from build123d import *

# Parameters (mm, degrees)
SKETCH1_W                  = 3
SKETCH1_H                  = 65
CUT_EXTRUDE1_DEPTH         = 66.138314378
CUT_EXTRUDE1_DEPTH_BACK    = 66.138314378
SKETCH2_R                  = 1.55
M3X0_5_TAPPED_HOLE1_REACH  = 67.138
M3X0_5_TAPPED_HOLE1_BORE_R = 1.25
CHAMFER1_SIZE              = 1
CHAMFER1_SIZE2             = 0.363970234


with BuildPart() as part:
    # Sketch1 → Revolve1 (revolve)
    with BuildSketch(Plane.XY, mode=Mode.PRIVATE) as revolve1_sk:
        with Locations((1.5, 32.5)):
            Rectangle(SKETCH1_W, SKETCH1_H)
    revolve(revolve1_sk.sketch.rotate(Axis((0, -5.428885746, 0), (0, 1, 0)), 90), axis=Axis((0, -5.428885746, 0), (0, 1, 0)))

    # Sketch2 → Cut-Extrude1 (cut, two sides: drawn at the far end of the back side and taken through both)
    with BuildSketch(Plane(origin=(0, 0, 0), x_dir=(0, 0, -1), z_dir=(1, 0, 0)).offset(-CUT_EXTRUDE1_DEPTH_BACK)):
        with Locations((0, 59)):
            Circle(SKETCH2_R)
    extrude(amount=CUT_EXTRUDE1_DEPTH + CUT_EXTRUDE1_DEPTH_BACK, mode=Mode.SUBTRACT)

    # M3x0.5 Tapped Hole1 bore → M3x0.5 Tapped Hole1 (cut, up to next)
    with BuildSketch(Plane(origin=(0, 65, 0), x_dir=(-1, 0, 0), z_dir=(0, 1, 0)), mode=Mode.PRIVATE) as m3x0_5_tapped_hole1_sk1:
        Circle(M3X0_5_TAPPED_HOLE1_BORE_R)
    m3x0_5_tapped_hole1_tool1 = extrude(m3x0_5_tapped_hole1_sk1.sketch, amount=-M3X0_5_TAPPED_HOLE1_REACH, mode=Mode.PRIVATE) & part.part
    add(m3x0_5_tapped_hole1_tool1.solids().sort_by_distance((0, 65, 0))[0], mode=Mode.SUBTRACT)

    # Chamfer1
    chamfer1_edges = [part.edges().sort_by_distance(p)[0] for p in [
        (0, 0, 3),
    ]]
    chamfer1_side = [part.faces().sort_by_distance(p)[0] for p in [
        (0, 32.5, 3),
    ]]
    chamfer(chamfer1_edges, length=CHAMFER1_SIZE, length2=CHAMFER1_SIZE2, reference=chamfer1_side[0])


solid = part.part
CAD build for the part. Positions are in the model's coordinates, mm. A direction names the side the tool comes from. Give positions to 0.01 mm unless a question says otherwise; leave off trailing zeros. Write each loop counter-clockwise with the first axis right and the second up, starting at its lowest first coordinate (ties: lowest second). Pieces come first, ordered by that corner, then holes. Notation, with made-up numbers: M -3,-23 L 32,-23 A19 ccw 32,7 Z; hole C 10.5,-22 d3. An arc over 180 degrees is marked long. Put each result on its own line as item: value. Start each with the question number.
(1) Probe L1, parallel to X at y = 60.9, z = 0; L2, parallel to Z at x = -0.25, y = 59; L3, parallel to Z at x = 1.25, y = 59. List the from-to ranges inside material, lowest first.
(2) Band-saw the part on C-C, the plane y = 59. Write the cut outline in (x, z), and give its area (3 significant figures).
(3) Which spindle directions (+Z, -Z, +X, -X, +Y, -Y) get a long thin tool onto all of the face, cutting with end or side? Do faces 1 (the face through (0, 0, 0)), 2 (the face through (-1.19, 62.49, 0.38)). Say none if no direction does.
(4) Band-saw the part on D-D, the plane y = 22.5. Write the cut outline in (x, z), and give its area (3 significant figures).
(5) Mould opens along Z. For faces 3 (the face through (-0.042, 57.487, 0.336)), 4 (the face through (1, 65, 1)), 5 (the face through (-0.9, 33.45, -2.86)) say: +Z half, -Z half, draft (parallel to the pull), parting line (faces both ways), or undercut.
(6) Band-saw the part on A-A, the plane z = 0. Write the cut outline in (x, y), and give its area (3 significant figures).
(7) Flat gauge pins, fed straight in: pin 1 Ø1.5 at (y, z) = (28.5, 1) entering from +X; pin 2 Ø2 at (x, y) = (-1.5, 18) entering from +Z. Where does each tip first touch, or does it go through?
(8) Band-saw the part on B-B, the plane x = 0. Write the cut outline in (y, z).
Response values:
1. L1: x = -3 to -1.25, 1.25 to 3
1. L2: z = -2.99 to -1.55, 1.55 to 2.99
1. L3: z = -2.73 to -1.55, 1.55 to 2.73
2. outline: M -2.57,-1.55 A3 ccw 2.57,-1.55 Z; M -2.57,1.55 L 2.57,1.55 A3 ccw Z
2. area: 10.5 mm2
3. face 1: +Z, -Z, +X, -X, -Y
3. face 2: +Y
4. outline: C 0,0 d6
4. area: 28.3 mm2
5. face 3: undercut
5. face 4: draft
5. face 5: parting line
6. outline: M -3,1 L -2.64,0 L 2.64,0 L 3,1 L 3,57.45 L -3,57.45 Z; M -3,60.55 L -1.25,60.55 L -1.25,65 L -3,65 Z; M 1.25,60.55 L 3,60.55 L 3,65 L 1.25,65 Z
6. area: 360 mm2
7. pin 1: stops at x = 2.99
7. pin 2: stops at z = 2.96
8. outline: M 0,-2.64 L 1,-3 L 65,-3 L 65,-1.25 L 59.92,-1.25 A1.55 cw long 59.92,1.25 L 65,1.25 L 65,3 L 1,3 L 0,2.64 Z
